Design review of the part built by this model. Coordinates are the model's own, in mm. Face numbers are marked on the shaded views. A direction names the side the tool comes from. Give positions to 0.01 mm unless a question says otherwise; leave off trailing zeros. Loops run counter-clockwise (first coordinate to the right, second up) from the corner with the lowest first, then second, coordinate; pieces in that order, holes last. Notation, with made-up numbers: (87, -13.5) -> (123, -13.5) arc R10 ccw to (123, -8.5) -> close; hole circle Ø6 at (-26.75, 55.25). An arc over 180 degrees is marked (long way). Use a Markdown table: item, result. Add a question column.
1. Add section B-B (x = 27). State the section outline as (y, z) points, and give its area (3 significant figures).
2. Add section A-A (z = -18). State the section outline as (x, y) points, and give its area (3 significant figures).
3. For the marked faces 1 and 2, list the 3-axis set-ups (+Z, -Z, +X, -X, +Y, -Y) from which the entire face can be reached by the end or side of a thin tool; tool diameter is ignored.
4. Add section D-D (x = 113.5). State the section outline as (y, z) points.
5. To check wall thickness, follow line 1 (Z direction, x = 50, y = 3); line 2 (Z direction, x = 95.5, y = 3.5); line 3 (X direction, y = 4.5, z = -71). State the ranges of each line that lie inside material, in increasing order.
6. Draft analysis for pull direction Z (two halves, no side actions). For the marked faces 3 and 4, state which applies: pulls with the +Z half, pulls with the -Z half, needs draft (parallel to the pull), parting line crosses it, or undercut.
7. Add section C-C (z = -72.5). State the section outline as (x, y) points.
8. For pin 1 Ø3.5 at (x, z) = (134, -24) entering from +Y; pin 2 Ø10 at (x, z) = (85, -12) entering from +Y, all flat-tipped, find the tip position at first contact; note any pin that passes through.
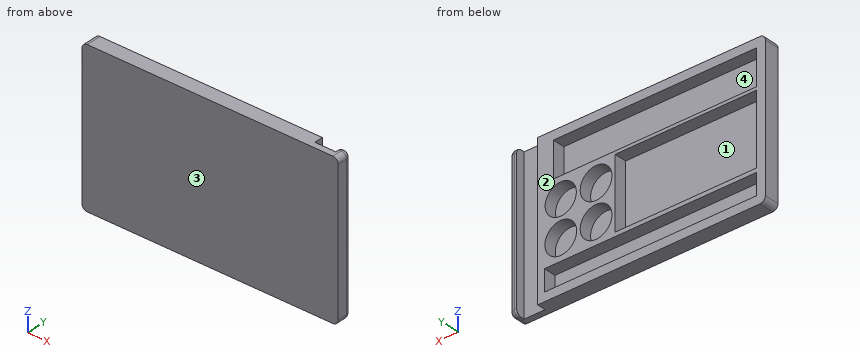
```python
from build123d import *

# Parameters (mm, degrees)
SKETCH_1_W            = 145
SKETCH_1_H            = 86
EXTRUDE_305_DEPTH     = 8.5
SKETCH_4_W            = 80
SKETCH_4_H            = 40
CUT_EXTRUDE_1_DEPTH   = 7
SKETCH_6_W            = 115
SKETCH_6_H            = 20
CUT_EXTRUDE_793_DEPTH = 7
SKETCH_8_W            = 120
SKETCH_8_H            = 12
CUT_EXTRUDE_5_DEPTH   = 7
SKETCH_14_R           = 9
SKETCH_14_R_2         = 8.831298305
CUT_EXTRUDE_11_DEPTH  = 7
SKETCH_15_W           = 11.88767394
SKETCH_15_H           = 86
CUT_EXTRUDE_12_DEPTH  = 5
FILLET_1_R            = 3
FILLET_2_R            = 3
FILLET_3_R            = 3
FILLET_4_R            = 3
FILLET_5_R            = 3


with BuildPart() as part:
    # Эскиз1 → Extrude 305 (new body)
    with BuildSketch(Plane(origin=(0, 0, 0), x_dir=(1, 0, 0), z_dir=(0, 1, 0))):
        with Locations((72.5, 43)):
            Rectangle(SKETCH_1_W, SKETCH_1_H)
    extrude(amount=EXTRUDE_305_DEPTH)

    # Эскиз4 → Вырез-Вытянуть1 (cut)
    with BuildSketch(Plane(origin=(0, 8.5, 0), x_dir=(1, 0, 0), z_dir=(0, 1, 0))):
        with Locations((45, 46.740912533)):
            Rectangle(SKETCH_4_W, SKETCH_4_H)
    extrude(amount=-CUT_EXTRUDE_1_DEPTH, mode=Mode.SUBTRACT)

    # Эскиз6 → Cut-Extrude 793 (cut)
    with BuildSketch(Plane(origin=(0, 8.5, 0), x_dir=(1, 0, 0), z_dir=(0, 1, 0))):
        with Locations((62.5, 15)):
            Rectangle(SKETCH_6_W, SKETCH_6_H)
    extrude(amount=-CUT_EXTRUDE_793_DEPTH, mode=Mode.SUBTRACT)

    # Эскиз8 → Вырез-Вытянуть5 (cut)
    with BuildSketch(Plane(origin=(0, 8.5, 0), x_dir=(1, 0, 0), z_dir=(0, 1, 0))):
        with Locations((65, 75)):
            Rectangle(SKETCH_8_W, SKETCH_8_H)
    extrude(amount=-CUT_EXTRUDE_5_DEPTH, mode=Mode.SUBTRACT)

    # Эскиз14 → Вырез-Вытянуть11 (cut)
    with BuildSketch(Plane(origin=(0, 8.5, 0), x_dir=(1, 0, 0), z_dir=(0, 1, 0))):
        with Locations((95.807220746, 36.975666029)):
            Circle(SKETCH_14_R)
        with Locations((115.807220746, 36.975666029)):
            Circle(SKETCH_14_R_2)
        with Locations((95.807220746, 56.975666029)):
            Circle(SKETCH_14_R)
        with Locations((115.807220746, 56.975666029)):
            Circle(SKETCH_14_R)
    extrude(amount=-CUT_EXTRUDE_11_DEPTH, mode=Mode.SUBTRACT)

    # Эскиз15 → Вырез-Вытянуть12 (cut)
    with BuildSketch(Plane(origin=(0, 8.5, 0), x_dir=(1, 0, 0), z_dir=(0, 1, 0))):
        with Locations((134.800217128, 43)):
            Rectangle(SKETCH_15_W, SKETCH_15_H)
    extrude(amount=-CUT_EXTRUDE_12_DEPTH, mode=Mode.SUBTRACT)

    # Скругление1
    fillet_1_edges = [part.edges().sort_by_distance(p)[0] for p in [
        (145, 8.5, -43),
    ]]
    fillet(fillet_1_edges, radius=FILLET_1_R)

    # Скругление2
    fillet_2_edges = [part.edges().sort_by_distance(p)[0] for p in [
        (145, 2.75, 0),
        (144.121320344, 7.621320344, 0),
        (141.372027049, 8.5, 0),
    ]]
    fillet(fillet_2_edges, radius=FILLET_2_R)

    # Скругление3
    fillet_3_edges = [part.edges().sort_by_distance(p)[0] for p in [
        (141.372027049, 8.5, -86),
        (145, 2.75, -86),
        (144.121320344, 7.621320344, -86),
    ]]
    fillet(fillet_3_edges, radius=FILLET_3_R)

    # Скругление4
    fillet_4_edges = [part.edges().sort_by_distance(p)[0] for p in [
        (0, 4.25, 0),
    ]]
    fillet(fillet_4_edges, radius=FILLET_4_R)

    # Скругление5
    fillet_5_edges = [part.edges().sort_by_distance(p)[0] for p in [
        (0, 4.25, -86),
    ]]
    fillet(fillet_5_edges, radius=FILLET_5_R)


solid = part.part
```
Taken from the geometry:
| question | item | result |
|---|---|---|
| 1 | outline | (0, -86) -> (8.5, -86) -> (8.5, -81) -> (1.5, -81) -> (1.5, -69) -> (8.5, -69) -> (8.5, -66.74) -> (1.5, -66.74) -> (1.5, -26.74) -> (8.5, -26.74) -> (8.5, -25) -> (1.5, -25) -> (1.5, -5) -> (8.5, -5) -> (8.5, 0) -> (0, 0) -> close |
| 1 | area | 227 mm^2 |
| 2 | outline | (0, 0) -> (145, 0) -> (145, 5.5) arc R3 ccw to (142, 8.5) -> (140.74, 8.5) -> (140.74, 3.5) -> (128.86, 3.5) -> (128.86, 8.5) -> (120, 8.5) -> (120, 1.5) -> (5, 1.5) -> (5, 8.5) -> (0, 8.5) -> close |
| 2 | area | 366 mm^2 |
| 3 | face 1 | +Y |
| 3 | face 2 | +Z, -Z, +X, -X, +Y |
| 4 | outline | (0, -86) -> (8.5, -86) -> (8.5, -81) -> (1.5, -81) -> (1.5, -69) -> (8.5, -69) -> (8.5, -65.67) -> (1.5, -65.67) -> (1.5, -48.28) -> (8.5, -48.28) -> (8.5, -45.5) -> (1.5, -45.5) -> (1.5, -28.45) -> (8.5, -28.45) -> (8.5, -25) -> (1.5, -25) -> (1.5, -5) -> (8.5, -5) -> (8.5, 0) -> (0, 0) -> close |
| 5 | line 1 | z = -86 to -81, -69 to -66.74, -26.74 to -25, -5 to 0 |
| 5 | line 2 | z = -86 to -81, -69 to -65.97, -47.98 to -45.97, -27.98 to -25, -5 to 0 |
| 5 | line 3 | x = 0 to 5, 125 to 128.86, 140.74 to 145 |
| 6 | face 3 | needs draft |
| 6 | face 4 | undercut |
| 7 | outline | (0, 0) -> (145, 0) -> (145, 5.5) arc R3 ccw to (142, 8.5) -> (140.74, 8.5) -> (140.74, 3.5) -> (128.86, 3.5) -> (128.86, 8.5) -> (125, 8.5) -> (125, 1.5) -> (5, 1.5) -> (5, 8.5) -> (0, 8.5) -> close |
| 8 | pin 1 | stops at y = 3.5 |
| 8 | pin 2 | stops at y = 1.5 |
